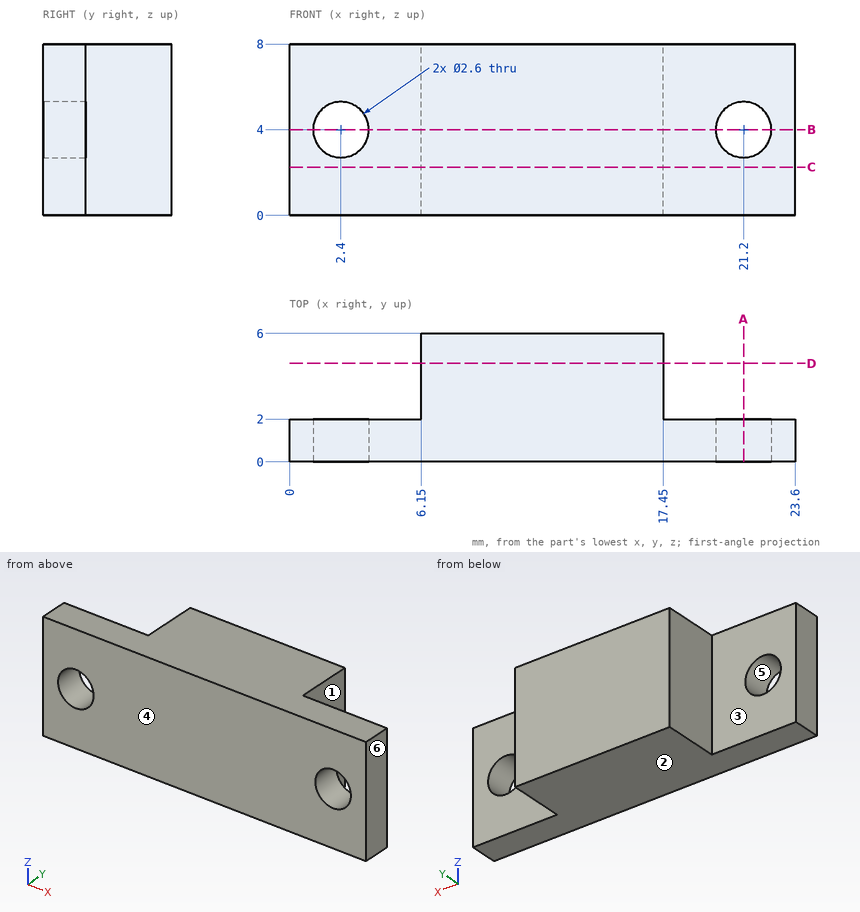
Print and shaded views of the part. All mm, measured from the part's lowest x, y and z. A direction names the side the tool comes from. Coordinates: 2 decimals unless noted, no trailing zeros. Loops run counter-clockwise (first coordinate to the right, second up) from the corner with the lowest first, then second, coordinate; pieces in that order, holes last. Notation, with made-up numbers: (-21.5, -5.75) - (-10.5, -5.75) arc R21 cw to (-10.5, 19.25) - close; hole circle Ø1 at (2, -27). An arc over 180 degrees is marked (long way). Write item = value, one per line. Start each with the question number.
Item 1: Cut at B-B, the plane z = 4. Give the cut face in (x, y), and give its area (3 significant figures).
Item 2: Cut at C-C, the plane z = 2.25. Give the cut face in (x, y).
Item 3: Mould opens along X. For the marked faces 4, 5 and 6 say: released by +X, released by -X, zero draft, split by the parting line, or undercut.
Item 4: Cut at A-A, the plane x = 21.2. Give the cut face in (y, z).
Item 5: Cut at D-D, the plane y = 4.6. Give the cut face in (x, z).
Item 6: Flat gauge pins, fed straight in: pin 1 Ø2.5 at (x, z) = (21.2, 4) entering from -Y; pin 2 Ø2 at (y, z) = (3.5, 2.5) entering from +X; pin 3 Ø3 at (x, z) = (3, 3) entering from +Y. Where does each tip first touch, or does it go through?
Item 7: 3-axis set-ups, long thin cutter, end or side, ignore diameter. For the marked faces 1, 2 and 3: which of +Z, -Z, +X, -X, +Y, -Y reach the whole face in a straight line?
Item 8: Wall check: L1, parallel to X at y = 0.95, z = 4; L2, parallel to Y at x = 17.75, z = 4.75; L3, parallel to X at y = 5.75, z = 7.5. Give the ranges that are in metal, low to high. Write a range as from..to.
The answers:
q1.outline = (0, 0) - (1.1, 0) - (1.1, 2) - (0, 2) - close; (3.7, 0) - (19.9, 0) - (19.9, 2) - (17.45, 2) - (17.45, 6) - (6.15, 6) - (6.15, 2) - (3.7, 2) - close; (22.5, 0) - (23.6, 0) - (23.6, 2) - (22.5, 2) - close
q1.area = 82.0 mm2
q2.outline = (0, 0) - (23.6, 0) - (23.6, 2) - (17.45, 2) - (17.45, 6) - (6.15, 6) - (6.15, 2) - (0, 2) - close
q3.face_4 = zero draft
q3.face_5 = undercut
q3.face_6 = released by +X
q4.outline = (0, 0) - (2, 0) - (2, 2.7) - (0, 2.7) - close; (0, 5.3) - (2, 5.3) - (2, 8) - (0, 8) - close
q5.outline = (6.15, 0) - (17.45, 0) - (17.45, 8) - (6.15, 8) - close
q6.pin_1 = through
q6.pin_2 = 17.45
q6.pin_3 = 2
q7.face_1 = +Z, -Z, +X, +Y
q7.face_2 = -Z, +X, -X, +Y, -Y
q7.face_3 = +Z, -Z, -X, +Y
q8.L1 = 0..1.1, 3.7..19.9, 22.5..23.6
q8.L2 = 0..2
q8.L3 = 6.15..17.45
